```python
from build123d import *
from build123d.topology import SkipClean

# Parameters (mm, degrees)
BOSS_EXTRUDE1_DEPTH       = 4.826
M3X0_5_TAPPED_HOLE2_D     = 2.5
M3X0_5_TAPPED_HOLE3_D     = 2.5
M3X0_5_TAPPED_HOLE3_DEPTH = 5
M3X0_5_TAPPED_HOLE3_TIP   = 0.751075774
FILLET1_R                 = 2.5
FILLET2_R                 = 4
SKETCH20_W                = 35
SKETCH20_H                = 4.826
SKETCH20_R                = 1.25
BOSS_EXTRUDE2_DEPTH       = 7


with BuildPart() as part:
    # Sketch1 → Boss-Extrude1 (new body)
    with BuildSketch(Plane.XY):
        Polygon((0, 0), (0, 13.5), (10, 13.5), (10, 20), (25, 20), (25, 7.5), (35, 7.5), (35, 0), align=None)
    extrude(amount=BOSS_EXTRUDE1_DEPTH)

    # M3x0.5 Tapped Hole2 (through all)
    with Locations(Plane.XY.offset(4.826)):
        with Locations((13.97024649, 12.44)):
            Hole(M3X0_5_TAPPED_HOLE2_D / 2)

    # M3x0.5 Tapped Hole3
    with Locations(Plane(origin=(0, 0, 0), x_dir=(-1, 0, 0), z_dir=(0, -1, 0))):
        with Locations((-16.73, -2.413), (-28.73, -2.413)):
            Hole(M3X0_5_TAPPED_HOLE3_D / 2, depth=M3X0_5_TAPPED_HOLE3_DEPTH)
            with Locations((0, 0, -(M3X0_5_TAPPED_HOLE3_DEPTH + M3X0_5_TAPPED_HOLE3_TIP / 2))):  # 118° drill point
                Cone(0, M3X0_5_TAPPED_HOLE3_D / 2, M3X0_5_TAPPED_HOLE3_TIP, mode=Mode.SUBTRACT)

    # Fillet1
    fillet1_edges = [part.edges().sort_by_distance(p)[0] for p in [
        (10, 20, 2.413),
        (10, 13.5, 2.413),
    ]]
    fillet(fillet1_edges, radius=FILLET1_R)

    # Fillet2
    fillet2_edges = [part.edges().sort_by_distance(p)[0] for p in [
        (25, 20, 2.413),
        (25, 7.5, 2.413),
        (35, 7.5, 2.413),
        (0, 13.5, 2.413),
    ]]
    fillet(fillet2_edges, radius=FILLET2_R)

    # Sketch20 → Boss-Extrude2 (add)
    with SkipClean():  # the faces are left unmerged after this step: merging them gives an invalid solid
        with BuildSketch(Plane.XZ):
            with Locations((17.5, 2.413)):
                Rectangle(SKETCH20_W, SKETCH20_H)
            with Locations(Location((28.73, 2.413, 0), (0, 0, 270))):
                Circle(SKETCH20_R, mode=Mode.SUBTRACT)
            with Locations(Location((16.73, 2.413, 0), (0, 0, 270))):
                Circle(SKETCH20_R, mode=Mode.SUBTRACT)
        extrude(amount=BOSS_EXTRUDE2_DEPTH)


solid = part.part
```
For this review, take the finished solid that the model builds, in its own axes (mm). A direction names the side the tool comes from. Round coordinates to 2 decimals unless told otherwise and drop trailing zeros. Write each loop counter-clockwise with the first axis right and the second up, starting at its lowest first coordinate (ties: lowest second). Pieces come first, ordered by that corner, then holes. Notation, with made-up numbers: (29, 10.25) - (59, 10.25) arc R22 cw to (59, 41.25) - close; hole circle Ø2 at (-5.75, 80.5). An arc over 180 degrees is marked (long way). Use CSV: the item, a comma, the result in double quotes.
1) Clearance check with flat-ended pins moving along their axes: pin 1 Ø1 at (x, z) = (30.5, 2.5) entering from +Y; pin 2 Ø2 at (x, z) = (28.73, 2.413) entering from -Y; pin 3 Ø1.2 at (y, z) = (16.5, 2) entering from -X; pin 4 Ø6 at (x, y) = (5.5, 14) entering from +Z. State where each tip first meets the part, or that it passes through.
Conclusion:
pin 1,"stops at y = 7.5"
pin 2,"stops at y = 5.15"
pin 3,"stops at x = 10"
pin 4,"stops at z = 4.83"
2) Add section A-A on y = 12.44. Write out the cut boundary in (x, z), and give its area (3 significant figures).
Conclusion:
outline,"(1.29, 0) - (12.72, 0) - (12.72, 4.83) - (1.29, 4.83) - close; (15.22, 0) - (25, 0) - (25, 4.83) - (15.22, 4.83) - close"
area,"102 mm^2"
3) The part is to be moulded in two halves that separate along X. For faces 1 (the conical face through (16.53, 5.62, 2.5)), 2 (the cylindrical face through (9, 14, 2)), 3 (the flat face through (30, 7.5, 2)), say which applies: pulls with the +X half, pulls with the -X half, needs draft (parallel to the pull), parting line crosses it, or undercut.
Conclusion:
face 1,"undercut"
face 2,"pulls with the -X half"
face 3,"needs draft"
4) Add section C-C on x = 10.5. Write out the cut boundary in (y, z).
Conclusion:
outline,"(-7, 0) - (19, 0) - (19, 4.83) - (-7, 4.83) - close"
5) For faces 4 (the flat face through (10, 17, 2)), 5 (the flat face through (17, 20, 2)), 6 (the flat face through (25, 14, 2)), list the 3-axis set-ups (+Z, -Z, +X, -X, +Y, -Y) from which the entire face can be reached by the end or side of a thin tool; tool diameter is ignored.
Conclusion:
face 4,"+Z, -Z, -X, +Y"
face 5,"+Z, -Z, +X, -X, +Y"
face 6,"+Z, -Z, +X, +Y"
6) Add section D-D on x = 3.5. Write out the cut boundary in (y, z), and give its area (3 significant figures).
Conclusion:
outline,"(-7, 0) - (13.47, 0) - (13.47, 4.83) - (-7, 4.83) - close"
area,"98.8 mm^2"
